```python
from build123d import *

# Parameters (mm, degrees)
SKETCH_1_W          = 48
SKETCH_1_H          = 15
EXTRUDE_1_DEPTH     = 6.5
SKETCH_2_W          = 22
SKETCH_2_H          = 15
EXTRUDE_2_DEPTH     = 20
FILLET_1_R          = 10
SKETCH_3_R          = 2.55
CUT_EXTRUDE_1_DEPTH = 34.700354834
SKETCH_4_R          = 5.25
SKETCH_4_R_2        = 1.55
CUT_EXTRUDE_2_DEPTH = 20
FILLET_2_R          = 2


with BuildPart() as part:
    # 草图1 → 凸台-拉伸1 (new body)
    with BuildSketch(Plane(origin=(0, 0, 0), x_dir=(1, 0, 0), z_dir=(0, 1, 0))):
        with Locations((-1.948504983, 0.398671096)):
            Rectangle(SKETCH_1_W, SKETCH_1_H)
    extrude(amount=EXTRUDE_1_DEPTH)

    # 草图2 → 凸台-拉伸2 (add)
    with BuildSketch(Plane(origin=(0, 6.5, 0), x_dir=(1, 0, 0), z_dir=(0, 1, 0))):
        with Locations((-1.948504983, 0.398671096)):
            Rectangle(SKETCH_2_W, SKETCH_2_H)
    extrude(amount=EXTRUDE_2_DEPTH)

    # 圆角1
    fillet_1_edges = [part.edges().sort_by_distance(p)[0] for p in [
        (-12.948504983, 26.5, -0.398671096),
        (9.051495017, 26.5, -0.398671096),
    ]]
    fillet(fillet_1_edges, radius=FILLET_1_R)

    # 草图3 → 切除-拉伸1 (cut, through all)
    with BuildSketch(Plane(origin=(0, 6.5, 0), x_dir=(1, 0, 0), z_dir=(0, 1, 0))):
        with Locations(Location((-19.948504983, 0.398671096, 0), (0, 0, 270))):
            Circle(SKETCH_3_R)
        with Locations(Location((16.051495017, 0, 0), (0, 0, 270))):
            Circle(SKETCH_3_R)
    extrude(amount=-CUT_EXTRUDE_1_DEPTH, mode=Mode.SUBTRACT)

    # 草图4 → 切除-拉伸2 (cut)
    with BuildSketch(Plane(origin=(0, 0, -7.898671096), x_dir=(-1, 0, 0), z_dir=(0, 0, -1))):
        with Locations((1.948504983, 14.5)):
            Circle(SKETCH_4_R)
        with Locations((1.948504983, 22.5)):
            Circle(SKETCH_4_R_2)
        with Locations((9.948504983, 14.5)):
            Circle(SKETCH_4_R_2)
        with Locations((1.948504983, 6.5)):
            Circle(SKETCH_4_R_2)
        with Locations((-6.051495017, 14.5)):
            Circle(SKETCH_4_R_2)
    extrude(amount=-CUT_EXTRUDE_2_DEPTH, mode=Mode.SUBTRACT)

    # 圆角2
    fillet_2_edges = [part.edges().sort_by_distance(p)[0] for p in [
        (-25.948504983, 3.25, -7.898671096),
        (22.051495017, 3.25, -7.898671096),
        (22.051495017, 3.25, 7.101328904),
        (-25.948504983, 3.25, 7.101328904),
    ]]
    fillet(fillet_2_edges, radius=FILLET_2_R)


solid = part.part
```
Verification items for the finished model (mm, model axes). A direction names the side the tool comes from. Coordinates: 2 decimals unless noted, no trailing zeros. Loops run counter-clockwise (first coordinate to the right, second up) from the corner with the lowest first, then second, coordinate; pieces in that order, holes last. Notation, with made-up numbers: (-28.75, -11) -> (-19.75, -11) arc R24 ccw to (-19.75, 27) -> close; hole circle Ø6 at (-7, 53). An arc over 180 degrees is marked (long way). Answer in a Markdown table with one row per item.
1) Draft check along X on faces 4 (the face through (21.45, 3.3, 6.53)), 5 (the face through (-7, 10, 7.101)), 6 (the face through (6.253, 16.037, -0.504)), 7 (the face through (-12.949, 11, 0)). Enter one of: released by +X, released by -X, zero draft, split by the parting line, or undercut.
The answers:
| item | result |
|---|---|
| face 4 | released by +X |
| face 5 | zero draft |
| face 6 | undercut |
| face 7 | released by -X |
2) Depth check by flat-ended pin: P1, Ø3, axis at y = 17, z = 0, coming from the +X side; P2, Ø6.5, axis at x = 15, z = -2.5, coming from the +Y side; P3, Ø2.5, axis at x = -1.95, y = 6.5, coming from the -Z side; P4, Ø8, axis at y = 12.5, z = -2, coming from the -X side. Enter the tip coordinate at first touch or a pass-through.
The answers:
| item | result |
|---|---|
| P1 | stops at x = 9.05 |
| P2 | stops at y = 6.5 |
| P3 | passes through |
| P4 | stops at x = -12.95 |
3) Section check C-C (z = 3.75). Record the cut outline in (x, y).
The answers:
| item | result |
|---|---|
| outline | (-25.95, 0) -> (22.05, 0) -> (22.05, 6.5) -> (9.05, 6.5) -> (9.05, 16.5) arc R10 ccw to (-0.95, 26.5) -> (-2.95, 26.5) arc R10 ccw to (-12.95, 16.5) -> (-12.95, 6.5) -> (-25.95, 6.5) -> close; hole circle Ø3.1 at (-9.95, 14.5); hole circle Ø10.5 at (-1.95, 14.5); hole circle Ø3.1 at (-1.95, 6.5); hole circle Ø3.1 at (-1.95, 22.5); hole circle Ø3.1 at (6.05, 14.5) |
4) Scan lines: line 1 along Y through (x, z) = (8, 1.25); line 2 along Y through (x, z) = (-13.5, -4); line 3 along Y through (x, z) = (-6.5, 2.25). Record each from-to range of solid material in increasing order. Write a range as from..to.
The answers:
| item | result |
|---|---|
| line 1 | y = 0..20.96 |
| line 2 | y = 0..6.5 |
| line 3 | y = 0..11.88, 17.12..25.85 |
5) Section check A-A (z = 0). Record the cut outline in (x, y), and give its area (3 significant figures).
The answers:
| item | result |
|---|---|
| outline | (-25.95, 0) -> (-22.47, 0) -> (-22.47, 6.5) -> (-25.95, 6.5) -> close; (-17.43, 0) -> (13.5, 0) -> (13.5, 6.5) -> (9.05, 6.5) -> (9.05, 16.5) arc R10 ccw to (-0.95, 26.5) -> (-2.95, 26.5) arc R10 ccw to (-12.95, 16.5) -> (-12.95, 6.5) -> (-17.43, 6.5) -> close; (18.6, 0) -> (22.05, 0) -> (22.05, 6.5) -> (18.6, 6.5) -> close; hole circle Ø3.1 at (-9.95, 14.5); hole circle Ø10.5 at (-1.95, 14.5); hole circle Ø3.1 at (-1.95, 6.5); hole circle Ø3.1 at (-1.95, 22.5); hole circle Ø3.1 at (6.05, 14.5) |
| area | 526 mm2 |
6) Access from +Z, -Z, +X, -X, +Y, -Y to the whole of each face (thin tool, end or side, straight path). Record for faces 1 (the face through (-17, 6.5, -1)), 2 (the face through (9.051, 11, 0)), 3 (the face through (-7, 10, -7.899)).
The answers:
| item | result |
|---|---|
| face 1 | +Z, -Z, -X, +Y |
| face 2 | +Z, -Z, +X, +Y |
| face 3 | -Z, +X, -X, +Y, -Y |
7) Section check B-B (y = 14.5). Record the cut outline in (x, z).
The answers:
| item | result |
|---|---|
| outline | (-12.95, -7.9) -> (-11.5, -7.9) -> (-11.5, 7.1) -> (-12.95, 7.1) -> close; (-8.4, -7.9) -> (-7.2, -7.9) -> (-7.2, 7.1) -> (-8.4, 7.1) -> close; (3.3, -7.9) -> (4.5, -7.9) -> (4.5, 7.1) -> (3.3, 7.1) -> close; (7.6, -7.9) -> (9.05, -7.9) -> (9.05, 7.1) -> (7.6, 7.1) -> close |
8) Section check D-D (y = 22.5). Record the cut outline in (x, z).
The answers:
| item | result |
|---|---|
| outline | (-10.95, -7.9) -> (-3.5, -7.9) -> (-3.5, 7.1) -> (-10.95, 7.1) -> close; (-0.4, -7.9) -> (7.05, -7.9) -> (7.05, 7.1) -> (-0.4, 7.1) -> close |
